For this review, take the finished solid that the model builds, in its own axes (mm). Face numbers are marked on the shaded views. Coordinates: 2 decimals unless noted, no trailing zeros. Loops run counter-clockwise (first coordinate to the right, second up) from the corner with the lowest first, then second, coordinate; pieces in that order, holes last. Notation, with made-up numbers: M 28,56.25 L 35,56.25 A20 ccw 35,89.25 Z; hole C 56.5,3.25 d7. An arc over 180 degrees is marked long. Write item = value, one per line.
from build123d import *

# Parameters (mm, degrees)
SKETCH1_R           = 10.5
BOSS_EXTRUDE1_DEPTH = 95
BOSS_EXTRUDE2_DEPTH = 1.5
SKETCH3_R           = 2.2
BOSS_EXTRUDE3_DEPTH = 9.4
BOSS_EXTRUDE3_TAPER = 1
SKETCH4_R           = 9.575
CUT_EXTRUDE1_DEPTH  = 93.5
SKETCH5_R           = 1
CUT_EXTRUDE2_DEPTH  = 107.471416352


with BuildPart() as part:
    # Sketch1 → Boss-Extrude1 (new body)
    with BuildSketch(Plane.XY):
        Circle(SKETCH1_R)
    extrude(amount=BOSS_EXTRUDE1_DEPTH)

    # Sketch2 → Boss-Extrude2 (add)
    with BuildSketch(Plane.XY.offset(95)):
        with BuildLine():
            Line((5.45, -11.8), (-5.45, -11.8))
            ThreePointArc((-5.45, -11.8), (-17.25, 0), (-5.45, 11.8))
            Line((-5.45, 11.8), (5.45, 11.8))
            ThreePointArc((5.45, 11.8), (17.25, 0), (5.45, -11.8))
        make_face()
    extrude(amount=-BOSS_EXTRUDE2_DEPTH)

    # Sketch3 → Boss-Extrude3 (add)
    with BuildSketch(Plane(origin=(0, 0, 0), x_dir=(-1, 0, 0), z_dir=(0, 0, -1))):
        with Locations((0, 6.5)):
            Circle(SKETCH3_R)
    extrude(amount=BOSS_EXTRUDE3_DEPTH, taper=BOSS_EXTRUDE3_TAPER)

    # Sketch4 → Cut-Extrude1 (cut)
    with BuildSketch(Plane.XY.offset(95)):
        Circle(SKETCH4_R)
    extrude(amount=-CUT_EXTRUDE1_DEPTH, mode=Mode.SUBTRACT)

    # Sketch5 → Cut-Extrude2 (cut, through all)
    with BuildSketch(Plane(origin=(0, 0, -9.4), x_dir=(-1, 0, 0), z_dir=(0, 0, -1))):
        with Locations((0, 6.5)):
            Circle(SKETCH5_R)
    extrude(amount=-CUT_EXTRUDE2_DEPTH, mode=Mode.SUBTRACT)


solid = part.part
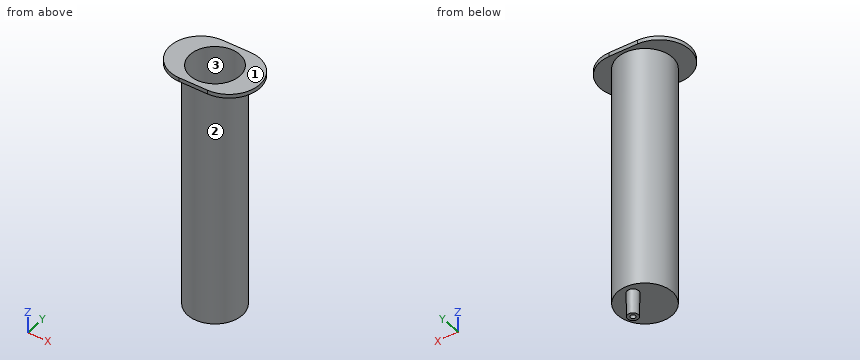
Q1. For pin 1 Ø3 at (y, z) = (8.5, 68.5) entering from +X; pin 2 Ø4 at (y, z) = (2.5, 70) entering from -X; pin 3 Ø6 at (x, y) = (-5.5, -0.5) entering from +Z; pin 4 Ø6 at (x, y) = (-1.5, 7) entering from +Z, all flat-tipped, find the tip position at first contact; note any pin that passes through.
Solved:
pin_1 = 7.83
pin_2 = -10.49
pin_3 = 1.5
pin_4 = 95
Q2. For line 1 along Y through (x, z) = (0, 63.5) (3 decimals); line 2 along X through (y, z) = (0.5, 69.5); line 3 along Z through (x, y) = (-7, 7.25), list the stretches that pass through material, from the lowest coordinate up.
Solved:
line_1 = -10.5 to -9.575, 9.575 to 10.5
line_2 = -10.49 to -9.56, 9.56 to 10.49
line_3 = 0 to 95
Q3. Add section D-D (x = 13). Write out the cut boundary in (y, z), and give its area (3 significant figures).
Solved:
outline = M -9.07,93.5 L 9.07,93.5 L 9.07,95 L -9.07,95 Z
area = 27.2 mm²
Q4. Add section C-C (x = -3.5). Write out the cut boundary in (y, z).
Solved:
outline = M -11.8,93.5 L -9.9,93.5 L -9.9,0 L 9.9,0 L 9.9,93.5 L 11.8,93.5 L 11.8,95 L 8.91,95 L 8.91,1.5 L -8.91,1.5 L -8.91,95 L -11.8,95 Z
Q5. Draft analysis for pull direction X (two halves, no side actions). For the marked faces 1, 2 and 3, state which applies: +X half, -X half, draft (parallel to the pull), parting line (faces both ways), or undercut.
Solved:
face_1 = draft
face_2 = parting line
face_3 = undercut
Q6. Add section A-A (y = 0). Write out the cut boundary in (x, z) (3 decimals).
Solved:
outline = M -17.25,93.5 L -10.5,93.5 L -10.5,0 L 10.5,0 L 10.5,93.5 L 17.25,93.5 L 17.25,95 L 9.575,95 L 9.575,1.5 L -9.575,1.5 L -9.575,95 L -17.25,95 Z
Q7. Add section B-B (z = 66). Write out the cut boundary in (x, y) (3 decimals), and give its area (3 significant figures).
Solved:
outline = C 0,0 d21; hole C 0,0 d19.15
area = 58.3 mm²
